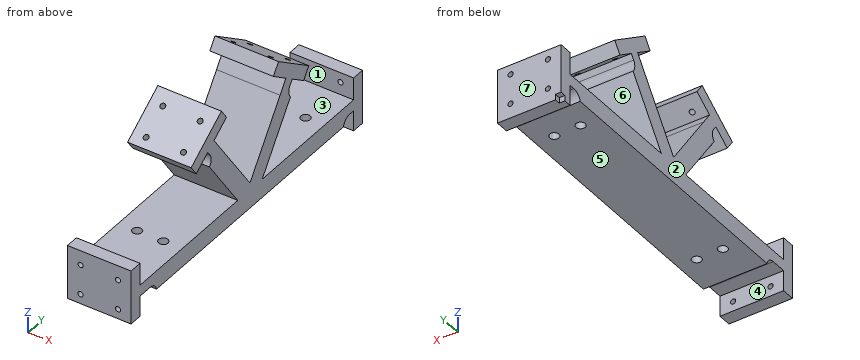
from build123d import *

# Parameters (mm, degrees)
SKETCH2_W           = 147.5
SKETCH2_H           = 176.75
BOSS_EXTRUDE1_DEPTH = 10
SKETCH3_W           = 29
SKETCH3_H           = 15
BOSS_EXTRUDE2_DEPTH = 34
BOSS_EXTRUDE3_DEPTH = 34
SKETCH8_W           = 113.5
SKETCH8_H           = 176.75
CUT_EXTRUDE1_DEPTH  = 30
SKETCH9_R           = 2.5
CUT_EXTRUDE2_DEPTH  = 134.016415209
SKETCH10_W          = 3
SKETCH10_H          = 3
CUT_EXTRUDE3_DEPTH  = 3
SKETCH11_R          = 1.4
CUT_EXTRUDE4_DEPTH  = 10
SKETCH12_R          = 1.4
CUT_EXTRUDE5_DEPTH  = 10
SKETCH13_R          = 1.4
CUT_EXTRUDE6_DEPTH  = 10
SKETCH14_R          = 1.4
CUT_EXTRUDE7_DEPTH  = 10
SKETCH15_W          = 11
SKETCH15_H          = 8
SKETCH15_W_2        = 12
CUT_EXTRUDE8_DEPTH  = 116.802867905
CUT_EXTRUDE9_DEPTH  = 116.802867905
FILLET1_R           = 5
BOSS_EXTRUDE4_START = 5
SKETCH17_W          = 34
SKETCH17_H          = 29
SKETCH17_R          = 1.4
BOSS_EXTRUDE4_DEPTH = 5
SKETCH18_W          = 11
SKETCH18_H          = 5
SKETCH18_W_2        = 12
CUT_EXTRUDE10_DEPTH = 120.662250585


with BuildPart() as part:
    # Sketch2 → Boss-Extrude1 (new body)
    with BuildSketch(Plane.XY):
        Rectangle(SKETCH2_W, SKETCH2_H)
    extrude(amount=BOSS_EXTRUDE1_DEPTH)

    # Sketch3 → Boss-Extrude2 (add)
    with BuildSketch(Plane.ZY.offset(73.75)):
        with Locations((7.5, 80.875)):
            Rectangle(SKETCH3_W, SKETCH3_H)
        with Locations((7.5, -80.875)):
            Rectangle(SKETCH3_W, SKETCH3_H)
    boss_extrude2 = extrude(amount=-BOSS_EXTRUDE2_DEPTH)

    # Mirror1: Boss-Extrude2 across plane
    add(boss_extrude2.mirror(Plane(origin=(0, 0, 0), x_dir=(0, 0, 1), z_dir=(1, 0, 0))))

    # Sketch5 → Boss-Extrude3 (add)
    with BuildSketch(Plane.ZY.offset(73.75)):
        Polygon((13.717233978, 0), (47.494362324, 23.650999887), (54.37727956, 13.821175356), (66.664560225, 22.424821901), (50.030843571, 46.180231185), (37.743562906, 37.57658464), (41.758597961, 31.84252033), (10, 9.604910635), (10, -9.604910635), (41.758597961, -31.84252033), (37.743562906, -37.57658464), (50.030843571, -46.180231185), (66.664560225, -22.424821901), (54.37727956, -13.821175356), (47.494362324, -23.650999887), align=None)
    extrude(amount=-BOSS_EXTRUDE3_DEPTH)

    # Sketch8 → Cut-Extrude1 (cut)
    with BuildSketch(Plane.XY.offset(22)):
        with Locations((17, 0)):
            Rectangle(SKETCH8_W, SKETCH8_H)
    extrude(amount=-CUT_EXTRUDE1_DEPTH, mode=Mode.SUBTRACT)

    # Sketch9 → Cut-Extrude2 (cut, through all)
    with BuildSketch(Plane(origin=(0, 0, 0), x_dir=(-1, 0, 0), z_dir=(0, 0, -1))):
        with Locations((49.75, 58.375)):
            Circle(SKETCH9_R)
        with Locations((63.75, 58.375)):
            Circle(SKETCH9_R)
        with Locations((49.75, -53.375)):
            Circle(SKETCH9_R)
        with Locations((63.75, -53.375)):
            Circle(SKETCH9_R)
    extrude(amount=-CUT_EXTRUDE2_DEPTH, mode=Mode.SUBTRACT)

    # Sketch10 → Cut-Extrude3 (cut)
    with BuildSketch(Plane(origin=(0, 0, -7), x_dir=(-1, 0, 0), z_dir=(0, 0, -1))):
        with Locations((72.25, 86.875)):
            Rectangle(SKETCH10_W, SKETCH10_H)
    extrude(amount=-CUT_EXTRUDE3_DEPTH, mode=Mode.SUBTRACT)

    # Sketch11 → Cut-Extrude4 (cut)
    with BuildSketch(Plane(origin=(0, 88.375, 0), x_dir=(1, 0, 0), z_dir=(0, 1, 0))):
        with Locations(Location((-46.75, -16.8, 0), (0, 0, 270))):
            Circle(SKETCH11_R)
        with Locations(Location((-66.75, -16.8, 0), (0, 0, 270))):
            Circle(SKETCH11_R)
        with Locations(Location((-66.75, -0.8, 0), (0, 0, 270))):
            Circle(SKETCH11_R)
        with Locations(Location((-46.75, -0.8, 0), (0, 0, 270))):
            Circle(SKETCH11_R)
    extrude(amount=-CUT_EXTRUDE4_DEPTH, mode=Mode.SUBTRACT)

    # Sketch12 → Cut-Extrude5 (cut)
    with BuildSketch(Plane.XZ.offset(88.375)):
        with Locations(Location((-46.75, -1.8, 0), (0, 0, 270))):
            Circle(SKETCH12_R)
        with Locations(Location((-66.75, -1.8, 0), (0, 0, 270))):
            Circle(SKETCH12_R)
        with Locations(Location((-66.75, 14.2, 0), (0, 0, 270))):
            Circle(SKETCH12_R)
        with Locations(Location((-46.75, 14.2, 0), (0, 0, 270))):
            Circle(SKETCH12_R)
    extrude(amount=-CUT_EXTRUDE5_DEPTH, mode=Mode.SUBTRACT)

    # Sketch13 → Cut-Extrude6 (cut)
    with BuildSketch(Plane(origin=(0, 38.699638206, 55.268811165), x_dir=(1, 0, 0), z_dir=(0, 0.5735764363510447, 0.8191520442889927))):
        with Locations(Location((-46.75, -14.667882182, 0), (0, 0, 270))):
            Circle(SKETCH13_R)
        with Locations(Location((-66.75, -14.667882182, 0), (0, 0, 270))):
            Circle(SKETCH13_R)
        with Locations(Location((-66.75, 1.332117818, 0), (0, 0, 270))):
            Circle(SKETCH13_R)
        with Locations(Location((-46.75, 1.332117818, 0), (0, 0, 270))):
            Circle(SKETCH13_R)
    extrude(amount=-CUT_EXTRUDE6_DEPTH, mode=Mode.SUBTRACT)

    # Sketch14 → Cut-Extrude7 (cut)
    with BuildSketch(Plane(origin=(0, -38.699638206, 55.268811165), x_dir=(1, 0, 0), z_dir=(0, -0.5735764363510447, 0.8191520442889929))):
        with Locations(Location((-46.75, -3.932117818, 0), (0, 0, 270))):
            Circle(SKETCH14_R)
        with Locations(Location((-66.75, -3.932117818, 0), (0, 0, 270))):
            Circle(SKETCH14_R)
        with Locations(Location((-66.75, 12.067882182, 0), (0, 0, 270))):
            Circle(SKETCH14_R)
        with Locations(Location((-46.75, 12.067882182, 0), (0, 0, 270))):
            Circle(SKETCH14_R)
    extrude(amount=-CUT_EXTRUDE7_DEPTH, mode=Mode.SUBTRACT)

    # Sketch15 → Cut-Extrude8 (cut, through all)
    with BuildSketch(Plane.ZY.offset(73.75)):
        with Locations((-1.5, 77.375)):
            Rectangle(SKETCH15_W, SKETCH15_H)
        with Locations((16, 77.375)):
            Rectangle(SKETCH15_W_2, SKETCH15_H)
        with Locations((16, -77.375)):
            Rectangle(SKETCH15_W_2, SKETCH15_H)
        with Locations((-1.5, -77.375)):
            Rectangle(SKETCH15_W, SKETCH15_H)
    extrude(amount=-CUT_EXTRUDE8_DEPTH, mode=Mode.SUBTRACT)

    # Sketch16 → Cut-Extrude9 (cut, through all)
    with BuildSketch(Plane.ZY.offset(73.75)):
        Polygon((37.743562906, 37.57658464), (41.758597961, 31.84252033), (44.052903706, 28.565912153), (50.60612006, 33.154523644), (44.296779261, 42.165196131), align=None)
        Polygon((54.047578679, 28.239611378), (47.494362324, 23.650999887), (54.37727956, 13.821175356), (60.930495915, 18.409786846), align=None)
        Polygon((47.494362324, -23.650999887), (54.047578679, -28.239611378), (60.930495915, -18.409786846), (54.37727956, -13.821175356), align=None)
        Polygon((37.743562906, -37.57658464), (44.296779261, -42.165196131), (50.60612006, -33.154523644), (44.052903706, -28.565912153), (41.758597961, -31.84252033), align=None)
    extrude(amount=-CUT_EXTRUDE9_DEPTH, mode=Mode.SUBTRACT)

    # Fillet1
    # the kernel refuses this fillet: 5 mm, written as the material it adds along each edge
    with BuildSketch(Plane(origin=(-73.75, -73.375, 4), x_dir=(0, -1, 0), z_dir=(1, 0, 0)), Plane(origin=(-73.75, -28.565912153, 44.052903706), x_dir=(0, -0.5735764363510428, 0.819152044288994), z_dir=(1, 0, 0))) as fillet1_piece_1:
        with BuildLine():
            CenterArc((4.898979486, 5), FILLET1_R, 191.536959033, 78.463040967)
            Line((0, 4), (-0.09797959, 3.98))
            ThreePointArc((-0.09797959, 3.98), (-0.1, 2), (-0.1, 0))
            Line((-0.1, 0), (0, -0.1))
            Line((0, -0.1), (4.898979486, -0.1))
            Line((4.898979486, -0.1), (4.898979486, 0))
        make_face()
    extrude(amount=34)
    with BuildSketch(Plane(origin=(-73.75, 28.565912153, 44.052903706), x_dir=(0, 0.8191520442898707, -0.5735764363497912), z_dir=(1, 0, 0))) as fillet1_piece_2:
        with BuildLine():
            CenterArc((5, 4.898979486), FILLET1_R, 180, 78.463040967)
            Line((0, 4.898979486), (-0.1, 4.898979486))
            Line((-0.1, 4.898979486), (-0.1, 0))
            Line((-0.1, 0), (0, -0.1))
            ThreePointArc((0, -0.1), (2, -0.1), (3.98, -0.09797959))
            Line((3.98, -0.09797959), (4, 0))
        make_face()
    extrude(amount=34)
    with BuildSketch(Plane(origin=(-73.75, 73.375, 4), x_dir=(0, 1, 0), z_dir=(1, 0, 0))) as fillet1_piece_3:
        with BuildLine():
            CenterArc((4.898979486, -5), FILLET1_R, 90, 78.463040967)
            Line((0, -4), (-0.09797959, -3.98))
            ThreePointArc((-0.09797959, -3.98), (-0.1, -2), (-0.1, 0))
            Line((-0.1, 0), (0, 0.1))
            Line((0, 0.1), (4.898979486, 0.1))
            Line((4.898979486, 0.1), (4.898979486, 0))
        make_face()
    extrude(amount=34)

    # Sketch17 → Boss-Extrude4 (add)
    with BuildSketch(Plane.XZ.offset(88.375).offset(BOSS_EXTRUDE4_START)):
        with Locations((-56.75, 7.5)):
            Rectangle(SKETCH17_W, SKETCH17_H)
        with Locations(Location((-66.75, 14.2, 0), (0, 0, 270))):
            Circle(SKETCH17_R, mode=Mode.SUBTRACT)
        with Locations(Location((-46.75, 14.2, 0), (0, 0, 270))):
            Circle(SKETCH17_R, mode=Mode.SUBTRACT)
        with Locations(Location((-46.75, -1.8, 0), (0, 0, 270))):
            Circle(SKETCH17_R, mode=Mode.SUBTRACT)
        with Locations(Location((-66.75, -1.8, 0), (0, 0, 270))):
            Circle(SKETCH17_R, mode=Mode.SUBTRACT)
    extrude(amount=-BOSS_EXTRUDE4_DEPTH)

    # Sketch18 → Cut-Extrude10 (cut, through all)
    with BuildSketch(Plane.ZY.offset(73.75)):
        with Locations((-1.5, -83.875)):
            Rectangle(SKETCH18_W, SKETCH18_H)
        with Locations((16, -83.875)):
            Rectangle(SKETCH18_W_2, SKETCH18_H)
    extrude(amount=-CUT_EXTRUDE10_DEPTH, mode=Mode.SUBTRACT)


solid = part.part
For this review, take the finished solid that the model builds, in its own axes (mm). Face numbers are marked on the shaded views. A direction names the side the tool comes from. Round coordinates to 2 decimals unless told otherwise and drop trailing zeros. Loops run counter-clockwise (first coordinate to the right, second up) from the corner with the lowest first, then second, coordinate; pieces in that order, holes last. Notation, with made-up numbers: (39.5, 5.5) - (59.5, 5.5) arc R19 cw to (59.5, 30.5) - close; hole circle Ø3 at (42.5, 7). An arc over 180 degrees is marked (long way). Use one line per item in the form item = value.
Item 1: Consider section C-C on x = -49.75. State how many separate pieces and enclosed holes the cut face has, then the cut area to 3 significant figures.
Answers:
separate_pieces = 3
enclosed_holes = 0
area = 3,260 mm^2
Item 2: Clearance check with flat-ended pins moving along their axes: P1, Ø0.9, axis at y = 86.5, z = -5.5, coming from the -X side; P2, Ø8, axis at x = -63.75, y = 58.375, coming from the -Z side; P3, Ø10, axis at x = -59, z = 28, coming from the -Y side; P4, Ø5, axis at y = -21.5, z = 19.5, coming from the +X side. State where each tip first meets the part, or that it passes through.
Answers:
P1 = -70.75
P2 = 0
P3 = -25.71
P4 = through
Item 3: For line 1 (X direction, y = 86, z = 0.8); line 2 (Z direction, x = -66.75, y = -88.5); line 3 (Z direction, x = -66, y = -88), list the stretches that pass through material, from the lowest coordinate up.
Answers:
line_1 = -73.75 to -68.15, -65.35 to -48.15, -45.35 to -39.75
line_2 = -7 to -3.2, -0.4 to 12.8, 15.6 to 22
line_3 = -7 to -2.98, -0.62 to 13.02, 15.38 to 22
Item 4: Tool access review of the marked faces 1, 2, 3 and 4: name each direction out of +Z, -Z, +X, -X, +Y, -Y from which nothing blocks a thin tool from reaching the whole face with its end or side.
Answers:
face_1 = +Z, +X, -X
face_2 = +Z, -Z, -X, +Y, -Y
face_3 = +X, -X
face_4 = -Z, +X, -X
Item 5: Consider section D-D on y = -48. Write out the cut boundary in (x, z).
Answers:
outline = (-73.75, 0) - (-39.75, 0) - (-39.75, 10) - (-73.75, 10) - close
Item 6: Consider section A-A on y = 16.5. Write out the cut boundary in (x, z).
Answers:
outline = (-73.75, 0) - (-39.75, 0) - (-39.75, 10) - (-73.75, 10) - close; (-73.75, 19.85) - (-39.75, 19.85) - (-39.75, 37.28) - (-73.75, 37.28) - close
Item 7: Consider section B-B on z = 39. Write out the cut boundary in (x, y).
Answers:
outline = (-73.75, -29.91) - (-39.75, -29.91) - (-39.75, -17.7) - (-73.75, -17.7) - close; (-73.75, 17.7) - (-39.75, 17.7) - (-39.75, 29.91) - (-73.75, 29.91) - close
Item 8: Mouldability with a two-part tool opening along Z and no side actions: class the marked faces 5, 6 and 7 as +Z half, -Z half, draft (parallel to the pull), parting line (faces both ways), or undercut.
Answers:
face_5 = -Z half
face_6 = undercut
face_7 = draft
